from build123d import *

# Parameters (mm, degrees)
SKETCH1_R           = 9.95
PISTON_DEPTH        = 5
SKETCH2_R           = 5
ROD_DEPTH           = 127
SKETCH3_W           = 81
SKETCH3_H           = 30
PLATE_DEPTH         = 10
SKETCH4_R           = 6
GUIDES_DEPTH        = 174.5
SKETCH5_R           = 1.5
MOUNTHOLES_DEPTH    = 6
CHAMFER1_SIZE       = 0.5
SKETCH6_R           = 2.5
MOUNTHOLES2_DEPTH   = 185.5
CUT_EXTRUDE1X_DEPTH = 3


with BuildPart() as part:
    # Sketch1 → Piston (new body)
    with BuildSketch(Plane.XY):
        Circle(SKETCH1_R)
    extrude(amount=PISTON_DEPTH)

    # Sketch2 → Rod (add)
    with BuildSketch(Plane.XY):
        Circle(SKETCH2_R)
    extrude(amount=ROD_DEPTH)

    # Sketch3 → Plate (add)
    with BuildSketch(Plane.XY.offset(127)):
        Rectangle(SKETCH3_W, SKETCH3_H)
    extrude(amount=PLATE_DEPTH)

    # Sketch4 → Guides (add)
    with BuildSketch(Plane(origin=(0, 0, 127), x_dir=(-1, 0, 0), z_dir=(0, 0, -1))):
        with Locations((-27, 0)):
            Circle(SKETCH4_R)
        with Locations((27, 0)):
            Circle(SKETCH4_R)
    extrude(amount=GUIDES_DEPTH)

    # Sketch5 → MountHoles (cut)
    with BuildSketch(Plane.XY.offset(137)):
        with Locations((14, 0)):
            Circle(SKETCH5_R)
        with Locations((-14, 0)):
            Circle(SKETCH5_R)
    extrude(amount=-MOUNTHOLES_DEPTH, mode=Mode.SUBTRACT)

    # Chamfer1
    chamfer1_edges = [part.edges().sort_by_distance(p)[0] for p in [
        (33, 0, -47.5),
        (-21, 0, -47.5),
    ]]
    chamfer(chamfer1_edges, length=CHAMFER1_SIZE)

    # Sketch6 → MountHoles2 (cut, through all)
    with BuildSketch(Plane.XY.offset(137)):
        with Locations((35, 9)):
            Circle(SKETCH6_R)
        with Locations((-35, 9)):
            Circle(SKETCH6_R)
        with Locations((35, -9)):
            Circle(SKETCH6_R)
        with Locations((-35, -9)):
            Circle(SKETCH6_R)
    extrude(amount=-MOUNTHOLES2_DEPTH, mode=Mode.SUBTRACT)

    # Sketch7 → Cut-Extrude1X (cut)
    with BuildSketch(Plane.XY.offset(137)):
        with BuildLine():
            Line((-14.25, 1.5), (-13.75, 1.5))
            ThreePointArc((-13.75, 1.5), (-12.25, 0), (-13.75, -1.5))
            Line((-13.75, -1.5), (-14.25, -1.5))
            ThreePointArc((-14.25, -1.5), (-15.75, 0), (-14.25, 1.5))
        make_face()
    extrude(amount=-CUT_EXTRUDE1X_DEPTH, mode=Mode.SUBTRACT)


solid = part.part
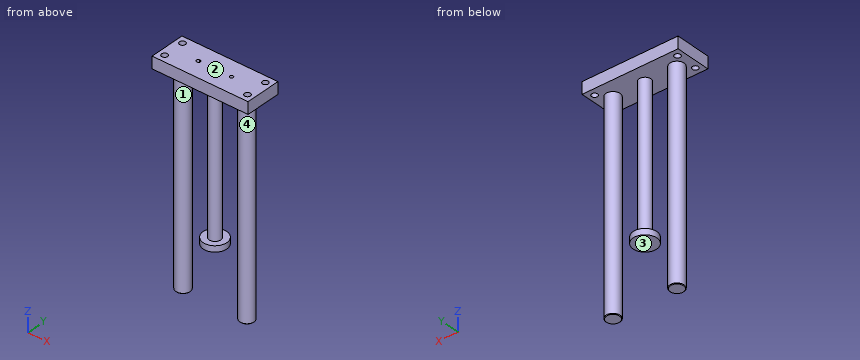
Can you work these out from the model? Positions are in its coordinate system, mm. Face numbers are marked on the shaded views. A direction names the side the tool comes from. Give positions to 0.01 mm unless a question says otherwise; leave off trailing zeros. Order: outer loops, then holes, each group sorted by start corner. A loop starts at its lowest first (then second) coordinate and runs counter-clockwise, first axis right, second up. Notation, with made-up numbers: M 89,75 L 106,75 A18 cw 106,84 Z; hole C 55,4 d6. An arc over 180 degrees is marked long. One line per question, with ' | ' between items.
Item 1: Suppose I cut it at A-A, the plane x = 27. Write out the boundary of the cut face in (y, z), then the cut area to 3 significant figures.
Answer block:
outline: M -15,127 L -6,127 L -6,-47 L -5.5,-47.5 L 5.5,-47.5 L 6,-47 L 6,127 L 15,127 L 15,137 L -15,137 Z | area: 2,390 mm2
Item 2: We'd pull the mould along X, two halves only. Please class the marked faces 1 and 2: released by +X, released by -X, zero draft, split by the parting line, or undercut.
Answer block:
face 1: undercut | face 2: zero draft
Item 3: Suppose I cut it at C-C, the plane z = 83. Write out the boundary of the cut face in (x, y), then the cut area to 3 significant figures.
Answer block:
outline: C -27,0 d12; C 0,0 d10; C 27,0 d12 | area: 305 mm2
Item 4: Please list where these lines run through material, in increasing order: L1, parallel to Y at x = -35, z = 130; L2, parallel to Z at x = -1, y = 8.75; L3, parallel to Y at x = 14, z = 133.9.
Answer block:
L1: y = -15 to -11.5, -6.5 to 6.5, 11.5 to 15 | L2: z = 0 to 5, 127 to 137 | L3: y = -15 to -1.5, 1.5 to 15
Item 5: Suppose I cut it at D-D, the plane x = 0. Write out the boundary of the cut face in (y, z).
Answer block:
outline: M -15,127 L -5,127 L -5,5 L -9.95,5 L -9.95,0 L 9.95,0 L 9.95,5 L 5,5 L 5,127 L 15,127 L 15,137 L -15,137 Z
Item 6: For the marked faces 3 and 4, which set-ups out of +Z, -Z, +X, -X, +Y, -Y let a thin tool reach every point of the face, with its end or its side?
Answer block:
face 3: -Z, +Y, -Y | face 4: -Z
Item 7: I'm going to push flat-ended pins straight in: pin 1 Ø1.4 at (x, y) = (-15, 0) entering from +Z; pin 2 Ø6 at (x, y) = (-17, 0) entering from -Z; pin 3 Ø8 at (y, z) = (4.5, 17) entering from -X; pin 4 Ø3 at (x, y) = (-35, -9) entering from -Z. Where does each tip first touch, or does it pass through?
Answer block:
pin 1: stops at z = 134 | pin 2: stops at z = 127 | pin 3: stops at x = -32.98 | pin 4: passes through
Item 8: Suppose I cut it at B-B, the plane x = -35. Write out the boundary of the cut face in (y, z).
Answer block:
outline: M -15,127 L -11.5,127 L -11.5,137 L -15,137 Z; M -6.5,127 L 6.5,127 L 6.5,137 L -6.5,137 Z; M 11.5,127 L 15,127 L 15,137 L 11.5,137 Z
